Can you work these out from the model? Positions are in its coordinate system, mm. A direction names the side the tool comes from. Coordinates: 2 decimals unless noted, no trailing zeros. Loops run counter-clockwise (first coordinate to the right, second up) from the corner with the lowest first, then second, coordinate; pieces in that order, holes last.
```python
from build123d import *

# Parameters (mm, degrees)
SKETCH1_R           = 1.324800001
SKETCH1_R_2         = 1.5
SKETCH1_W           = 6.35
SKETCH1_H           = 3.175
BOSS_EXTRUDE1_DEPTH = 3.175


with BuildPart() as part:
    # Sketch1 → Boss-Extrude1 (new body)
    with BuildSketch(Plane(origin=(0, 0, 0), x_dir=(1, 0, 0), z_dir=(0, 1, 0))):
        with BuildLine():
            Line((241.90748173, 29.781172289), (266.90748173, 29.781172289))
            ThreePointArc((266.90748173, 29.781172289), (270.443015636, 28.316706195), (271.90748173, 24.781172289))
            Line((271.90748173, 24.781172289), (271.90748173, -34.394734405))
            ThreePointArc((271.90748173, -34.394734405), (270.443015636, -37.930268311), (266.90748173, -39.394734405))
            Line((266.90748173, -39.394734405), (241.90748173, -39.394734405))
            ThreePointArc((241.90748173, -39.394734405), (238.371947824, -37.930268311), (236.90748173, -34.394734405))
            Line((236.90748173, -34.394734405), (236.90748173, 24.781172289))
            ThreePointArc((236.90748173, 24.781172289), (238.371947824, 28.316706195), (241.90748173, 29.781172289))
        make_face()
        with Locations(Location((254.350862197, 24.256669994, 0), (0, 0, 270))):
            Circle(SKETCH1_R, mode=Mode.SUBTRACT)
        with Locations(Location((249.226245104, 5.131338633, 0), (0, 0, 90))):
            Circle(SKETCH1_R, mode=Mode.SUBTRACT)
        with Locations(Location((249.226245104, -14.744900749, 0), (0, 0, 270))):
            Circle(SKETCH1_R, mode=Mode.SUBTRACT)
        with Locations(Location((254.350862197, -33.870232109, 0), (0, 0, 90))):
            Circle(SKETCH1_R, mode=Mode.SUBTRACT)
        with Locations(Location((254.40748173, -4.806781058, 0), (0, 0, 270))):
            Circle(SKETCH1_R_2, mode=Mode.SUBTRACT)
        Polygon((240.775666346, 11.14605698), (262.991960351, 5.193218942), (266.241381147, 17.32022245), (244.025087143, 23.273060488), align=None, mode=Mode.SUBTRACT)
        Polygon((262.991960351, -14.806781058), (266.241381147, -26.933784566), (244.025087143, -32.886622603), (240.775666346, -20.759619095), align=None, mode=Mode.SUBTRACT)
        with Locations((246.43248173, -4.806781058)):
            Rectangle(SKETCH1_W, SKETCH1_H, mode=Mode.SUBTRACT)
        with Locations((262.38248173, -4.806781058)):
            Rectangle(SKETCH1_W, SKETCH1_H, mode=Mode.SUBTRACT)
    extrude(amount=BOSS_EXTRUDE1_DEPTH)


solid = part.part
```
(1) If I drill on probe 1 along Z at (x, y) = (258, 0.9); probe 2 along Z at (x, y) = (260, 0.95); probe 3 along X at (y, z) = (1.6, 3.5), over which ranges is the centre line in solid material (lowest first)?
Check values:
probe 1: z = -29.78 to -19.53, -6.53 to 16.14, 29.14 to 39.39
probe 2: z = -29.78 to -18.99, -5.99 to 3.22, 6.39 to 15.61, 28.61 to 39.39
probe 3: x = 236.91 to 243.26, 249.61 to 253.67, 255.14 to 259.21, 265.56 to 271.91
(2) I want a section at D-D on y = 2.1. State how many separate pieces and enclosed holes the cut face has, then the cut area to 3 significant figures.
Check values:
separate pieces: 1
enclosed holes: 9
area: 1,750 mm2
(3) I want a section at C-C on x = 257.5. Write out the boundary of the cut face in (y, z) (3 decimals), then the cut area to 3 significant figures.
Check values:
outline: (0, -29.781) - (3.175, -29.781) - (3.175, -19.662) - (0, -19.662) - close; (0, -6.665) - (3.175, -6.665) - (3.175, 16.278) - (0, 16.278) - close; (0, 29.276) - (3.175, 29.276) - (3.175, 39.395) - (0, 39.395) - close
area: 137 mm2
(4) I want a section at B-B on x = 264.5. Write out the boundary of the cut face in (y, z) (3 decimals), then the cut area to 3 significant figures.
Check values:
outline: (0, -29.781) - (3.175, -29.781) - (3.175, -17.787) - (0, -17.787) - close; (0, -10.821) - (3.175, -10.821) - (3.175, 3.219) - (0, 3.219) - close; (0, 6.394) - (3.175, 6.394) - (3.175, 20.435) - (0, 20.435) - close; (0, 27.4) - (3.175, 27.4) - (3.175, 39.395) - (0, 39.395) - close
area: 165 mm2
(5) If we mould it in two halves opening along Z, with no side actions, what happens to faces 1 (the flat face through (259.207, 2, 5)), 2 (the cylindrical face through (270.4, 1.57, -28.36)), 3 (the flat face through (236.907, 2, 5))? For each: released by +Z, released by -Z, zero draft, split by the parting line, or undercut.
Check values:
face 1: undercut
face 2: released by -Z
face 3: zero draft
(6) Which directions (+Z, -Z, +X, -X, +Y, -Y) give clear straight access to the entire face, cutting with the end or side of a thin tool? Please do faces 4 (the flat face through (242.42, 1.57, -17.29)), 5 (the cylindrical face through (270.482, 1.565, 37.891)).
Check values:
face 4: +Y, -Y
face 5: +Z, +X, +Y, -Y
(7) I'm going to push flat-ended pins straight in: pin 1 (1.6 mm diameter, centred on x = 249.23, z = 14.74, fed in from -Y); pin 2 (1 mm diameter, centred on x = 240.5, y = 0.5, fed in from -Z). Where does each tip first touch, or does it pass through?
Check values:
pin 1: passes through
pin 2: stops at z = -29.7
(8) I want a section at A-A on z = 25.5. Write out the boundary of the cut face in (x, y) (3 decimals), then the cut area to 3 significant figures.
Check values:
outline: (236.907, 0) - (242.046, 0) - (242.046, 3.175) - (236.907, 3.175) - close; (265.857, 0) - (271.907, 0) - (271.907, 3.175) - (265.857, 3.175) - close
area: 35.5 mm2
